Autodesk Inventor part; units mm, degrees
ref_plane "YZ Plane" through (0, 0, 0) normal (1, 0, 0) x (0, 1, 0)
ref_plane "XZ Plane" through (0, 0, 0) normal (0, 1, 0) x (-1, 0, 0)
ref_plane "XY Plane" through (0, 0, 0) normal (0, 0, 1) x (1, 0, 0)
ref_plane "Work Plane1" through (0, 0, 0) normal (0, 0, 1) x (1, 0, 0)
sketch "Sketch1" plane through (0, 0, 0) normal (0, 0, 1) x (1, 0, 0)
  line L0 (372.5286, -363.5164) -> (372.5286, 136.4836)
  line L1 (372.5286, 136.4836) -> (225.6417, 451.4836)
  line L2 (225.6417, 451.4836) -> (-104.3583, 451.4836) construction
  line L3 (-185.3519, -363.5164) -> (372.5286, -363.5164) construction
  line L4 (225.6417, 451.4836) -> (60.6417, 451.4836)
  line L5 (60.6417, 401.4836) -> (60.6417, 451.4836)
  line L6 (372.5286, -363.5164) -> (60.6417, -363.5164)
  line L7 (60.6417, 401.4836) -> (60.6417, -363.5164) construction
  line L8 (59.0417, 453.0836) -> (226.661, 453.0836)
  line L9 (226.661, 453.0836) -> (374.1286, 136.8383)
  line L10 (374.1286, 136.8383) -> (374.1286, -365.1164)
  line L11 (374.1286, -365.1164) -> (60.6417, -365.1164)
  line L12 (60.6417, -363.5164) -> (60.6417, -365.1164)
  line L13 (60.6417, 401.4836) -> (59.0417, 401.4836)
  line L14 (59.0417, 401.4836) -> (59.0417, 453.0836)
  point P0 (0, 0)
  dimension "d0" = 50
  dimension "d1" = 1.6
  dimension "d2" = 1.6
  dimension "d3" = 816.6
  dimension "d4" = 816.6
extrude "Extrusion1" add sketch "Sketch1" along normal blind 1198.4 and the other way blind 1.6
sketch "Sketch2" plane through (59.0417, 401.4836, -1.6) normal (-1, 0, 0) x (0, 0, 1)
  line L0 (0, 0) -> (0, 51.6)
  line L1 (1200, 0) -> (0, 0)
  line L2 (0, 50) -> (0, 0)
  line L3 (0, 0) -> (1.6, 0)
  line L4 (1.6, 0) -> (1.6, 50)
  line L5 (0, 50) -> (1.6, 50)
  point P0 (1.6, -401.4836)
  point P1 (0, 50)
  dimension "d14" = 1.6
extrude "Extrusion2" cut sketch "Sketch2" against normal blind 1.6
ref_plane "Work Plane2" through (0, 0, 598.4) normal (0, 0, 1) x (1, 0, 0)
mirror "Mirror1" about plane through (0, 0, 598.4) normal (0, 0, 1) of "Extrusion2"
properties part number "Back Cover"
Work out the finished part from the listing and answer in its coordinate system (mm). A direction names the side the tool comes from. Coordinates: 2 decimals unless noted, no trailing zeros. Order: outer loops, then holes, each group sorted by start corner. A loop starts at its lowest first (then second) coordinate and runs counter-clockwise, first axis right, second up. Notation, with made-up numbers: (36, -0.5) - (48, -0.5) arc R21 ccw to (48, 19.5) - close; hole circle Ø3 at (16.5, 62.5). An arc over 180 degrees is marked (long way). Answer as a JSON object with one key per item and string values.
1. Each of these flat-tipped pins is pushed along its axis until it touches: P1, Ø5, axis at x = 299, z = 154.5, coming from the +Y side; P2, Ø0.8, axis at x = 60, z = 658.5, coming from the -Y side; P3, Ø15, axis at y = 439, z = 552, coming from the +X side. Where does it stop, or does it pass through?
Output values:
{"P1": "stops at y = 303.31", "P2": "stops at y = 401.48", "P3": "stops at x = 236.73"}
2. The mould has two halves that part along X. Classify faces 1 (the face through (372.529, -117, 590)), 2 (the face through (60.642, 426, 590)), 3 (the face through (299.363, 297.175, 590)): +X half, -X half, draft (parallel to the pull), parting line (faces both ways), or undercut.
Output values:
{"face 1": "-X half", "face 2": "undercut", "face 3": "+X half"}
3. A tool of negligible diameter and unlimited length cuts with its end or side. For faces 4 (the face through (220, -365.116, 590)), 5 (the face through (219, -363.516, 590)), 6 (the face through (144, 451.484, 590)), from which of +Z, -Z, +X, -X, +Y, -Y can it reach the whole face along a straight path? Write none if from no direction.
Output values:
{"face 4": "+Z, -Z, +X, -X, -Y", "face 5": "+Z, -Z, -X", "face 6": "+Z, -Z"}
4. Find section D-D on y = 17. Determine the outline of the cut face in (x, z).
Output values:
{"outline": "(372.53, -1.6) - (374.13, -1.6) - (374.13, 1198.4) - (372.53, 1198.4) - close"}
5. Find section A-A on x = 139. Determine the outline of the cut face in (y, z), plus the area to 3 significant figures.
Output values:
{"outline": "(-365.12, -1.6) - (-363.52, -1.6) - (-363.52, 1198.4) - (-365.12, 1198.4) - close; (451.48, -1.6) - (453.08, -1.6) - (453.08, 1198.4) - (451.48, 1198.4) - close", "area": "3,840 mm²"}
6. Consider line 1 (Y direction, x = 107, z = 1035); line 2 (Y direction, x = 316.5, z = 494.5); line 3 (X direction, y = -178, z = 1125.5). Determine where each line is inside the solid, lowest interval first.
Output values:
{"line 1": "y = -365.12 to -363.52, 451.48 to 453.08", "line 2": "y = -365.12 to -363.52, 256.64 to 260.42", "line 3": "x = 372.53 to 374.13"}
7. Find section C-C on x = 321. Determine the outline of the cut face in (y, z), plus the area to 3 significant figures.
Output values:
{"outline": "(-365.12, -1.6) - (-363.52, -1.6) - (-363.52, 1198.4) - (-365.12, 1198.4) - close; (246.99, -1.6) - (250.77, -1.6) - (250.77, 1198.4) - (246.99, 1198.4) - close", "area": "6,460 mm²"}
8. Find section B-B on z = 1071. Determine the outline of the cut face in (x, y).
Output values:
{"outline": "(59.04, 401.48) - (60.64, 401.48) - (60.64, 451.48) - (225.64, 451.48) - (372.53, 136.48) - (372.53, -363.52) - (60.64, -363.52) - (60.64, -365.12) - (374.13, -365.12) - (374.13, 136.84) - (226.66, 453.08) - (59.04, 453.08) - close"}
